Work out the finished part from the listing and answer in its coordinate system (mm). A direction names the side the tool comes from. Give positions to 0.01 mm unless a question says otherwise; leave off trailing zeros. Write each loop counter-clockwise with the first axis right and the second up, starting at its lowest first coordinate (ties: lowest second). Pieces come first, ordered by that corner, then holes.
1) Straight lines are drawn through the part: probe 1 along Z at (x, y) = (0, 7.5); probe 2 along Y at (x, z) = (-0.7, -3.05); probe 3 along Y at (x, z) = (-1.1, -0.4). For each, find the intervals that lie inside material, in ascending order.
2) Find section C-C (y = -1). Determine the outline of the cut face in (x, z), plus the area to 4 significant figures.
3) Find section B-B (z = -3.85). Determine the outline of the cut face in (x, y), plus the area to 3 significant figures.
4) Find section A-A (x = 0). Determine the outline of the cut face in (y, z), plus the area to 3 significant figures.
5) Given pin 1 Ø1.5 at (x, y) = (1, 9) entering from -Z, flat-ended and moving along its own axis, determine where the tip first touches the part or whether it passes through.
6) A tool of negligible diameter and unlimited length cuts with its end or side. For faces 1 (the face through (0, 7, -3)), 2 (the face through (1.22, -1.04, -2.22)), from which of +Z, -Z, +X, -X, +Y, -Y can it reach the whole face along a straight path? Write none if from no direction.
7) Find section D-D (z = -1.7). Determine the outline of the cut face in (x, y).
```python
from build123d import *

# Parameters (mm, degrees)
EXTRUDE_1_DEPTH          = 4.5
EXTRUDE_2_DEPTH          = 5
SKETCH_4_W               = 4.107505073
SKETCH_4_H               = 2.274071006
CUT_EXTRUDE_1_DEPTH      = 13
CUT_EXTRUDE_1_DEPTH_BACK = 3
FILLET_1_R               = 1
FILLET_2_R               = 0.5


with BuildPart() as part:
    # Эскиз1 → Бобышка-Вытянуть1 (new body)
    with BuildSketch(Plane.XY):
        Polygon((2, 0), (2, 5), (-2, 5), (-2, 0), (-0.5, -2), (0.5, -2), align=None)
    extrude(amount=-EXTRUDE_1_DEPTH)

    # Эскиз2 → Бобышка-Вытянуть2 (add)
    with BuildSketch(Plane(origin=(0, 5, 0), x_dir=(1, 0, 0), z_dir=(0, 1, 0))):
        with BuildLine():
            Line((-1.732050808, 0), (1.732050808, 0))
            ThreePointArc((1.732050808, 0), (0, 3), (-1.732050808, 0))
        make_face()
    extrude(amount=EXTRUDE_2_DEPTH)

    # Эскиз3 → Повернуть1 (revolve)
    with BuildSketch(Plane(origin=(0, 10, 0), x_dir=(1, 0, 0), z_dir=(0, 1, 0))):
        with BuildLine():
            ThreePointArc((2, 1), (0, 3), (-2, 1))
            Line((-2, 1), (2, 1))
        make_face()
    revolve(axis=Axis((-2, 10, -1), (1, 0, 0)))

    # Эскиз4 → Вырез-Вытянуть1 (cut, two sides)
    with BuildSketch(Plane(origin=(0, 0, 0), x_dir=(1, 0, 0), z_dir=(0, 1, 0))) as cut_extrude_1_sk:
        with Locations((0.053752537, -1.137035503)):
            Rectangle(SKETCH_4_W, SKETCH_4_H)
    extrude(amount=CUT_EXTRUDE_1_DEPTH, mode=Mode.SUBTRACT)
    extrude(cut_extrude_1_sk.sketch, amount=-CUT_EXTRUDE_1_DEPTH_BACK, mode=Mode.SUBTRACT)

    # Скругление1
    fillet_1_edges = [part.edges().sort_by_distance(p)[0] for p in [
        (2, 0, -2.25),
        (-2, 0, -2.25),
    ]]
    fillet(fillet_1_edges, radius=FILLET_1_R)

    # Скругление2
    fillet_2_edges = [part.edges().sort_by_distance(p)[0] for p in [
        (0.5, -2, -2.25),
        (-0.5, -2, -2.25),
    ]]
    fillet(fillet_2_edges, radius=FILLET_2_R)


solid = part.part
```
Results:
1. probe 1: z = -3 to 0
1. probe 2: y = -1.73 to 5
1. probe 3: y = -1.2 to 11.56
2. outline: (-1.25, -4.5) - (1.25, -4.5) - (1.25, 0) - (-1.25, 0) - close
2. area: 11.25 mm2
3. outline: (-2, 0.33) arc R1 ccw to (-1.8, -0.27) - (-0.65, -1.8) arc R0.5 ccw to (-0.25, -2) - (0.25, -2) arc R0.5 ccw to (0.65, -1.8) - (1.8, -0.27) arc R1 ccw to (2, 0.33) - (2, 5) - (-2, 5) - close
3. area: 25.0 mm2
4. outline: (-2, -4.5) - (5, -4.5) - (5, -3) - (10, -3) arc R2 ccw to (11.73, 0) - (-2, 0) - close
4. area: 51.6 mm2
5. pin 1: stops at z = -2.98
6. face 1: +Y
6. face 2: +Z, -Z, +X, -Y
7. outline: (-2, 0.33) arc R1 ccw to (-1.8, -0.27) - (-0.65, -1.8) arc R0.5 ccw to (-0.25, -2) - (0.25, -2) arc R0.5 ccw to (0.65, -1.8) - (1.8, -0.27) arc R1 ccw to (2, 0.33) - (2, 5) - (1.87, 5) - (1.87, 10) arc R1.87 ccw to (-1.87, 10) - (-1.87, 5) - (-2, 5) - close
